Read the model definition and answer for the solid it produces. Units are mm, in the model's axes. Give positions to 0.01 mm unless a question says otherwise; leave off trailing zeros. Write each loop counter-clockwise with the first axis right and the second up, starting at its lowest first coordinate (ties: lowest second). Pieces come first, ordered by that corner, then holes.
Autodesk Fusion 360 part; units mm, degrees
sketch "Sketch1" plane through (0, 0, 0) normal (0, 0, 1) x (1, 0, 0)
  line L0 (-64.0556, -47.9598) -> (-64.1923, -47.777)
  line L1 (-64.0556, -47.9598) -> (-63.9189, -48.1426)
  arc A0 (-64.1923, -47.777) -> (-57.1589, -48.7607) centre (-60.188, -44.7827) ccw
  arc A1 (-62.8738, -41.1181) -> (-63.9189, -48.1426) centre (-59.9146, -45.1483) ccw
  line L2 (-49.93, 3.9993) -> (0.06, 2.9994)
  line L3 (-0.06, -2.9994) -> (-50.05, -1.9996)
  arc A2 (-49.93, 3.9993) -> (-50.05, -1.9996) centre (-49.99, 0.9998) ccw
  arc A3 (-0.06, -2.9994) -> (0.06, 2.9994) centre (0, 0) ccw
  circle A4 centre (0, 0) radius 1
  point P0 (-4, 4.6)
  dimension "d2" = 5
  dimension "d3" = 5
  dimension "d10" = 6
  dimension "d11" = 6
  dimension "d13" = 50
  dimension "d14" = 2
extrude "Extrude2" add sketch "Sketch1" along normal blind 1 contours L2 L3 A2 A3
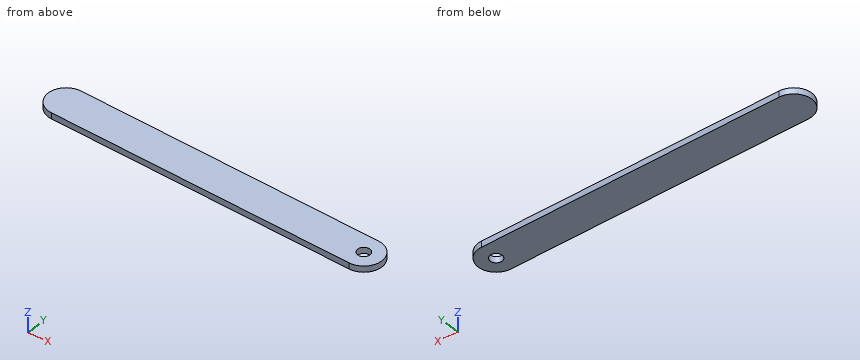
Item 1: Section A-A (y = 0) is taken. Write down the section's boundary in (x, z), and give its area (3 significant figures).
Result set:
outline: (-52.82, 0) - (-1, 0) - (-1, 1) - (-52.82, 1) - close; (1, 0) - (3, 0) - (3, 1) - (1, 1) - close
area: 53.8 mm2
Item 2: Section B-B (z = 0.4) is taken. Write down the section's boundary in (x, y).
Result set:
outline: (-50.05, -2) - (-0.06, -3) arc R3 ccw to (0.06, 3) - (-49.93, 4) arc R3 ccw to start; hole circle Ø2 at (0, 0)
Item 3: Section C-C (x = -10) is taken. Write down the section's boundary in (y, z).
Result set:
outline: (-2.8, 0) - (3.2, 0) - (3.2, 1) - (-2.8, 1) - close
Item 4: Find the intervals of material crossed by line 1 along Y through (x, z) = (0, 0.45); line 2 along X through (y, z) = (-0.25, 0.65); line 3 along X through (y, z) = (1.25, 0.6), in increasing order.
Result set:
line 1: y = -3 to -1, 1 to 3
line 2: x = -52.72 to -0.97, 0.97 to 2.99
line 3: x = -52.98 to 2.73
